Verification items for the finished model (mm, model axes). A direction names the side the tool comes from. Coordinates: 2 decimals unless noted, no trailing zeros. Write each loop counter-clockwise with the first axis right and the second up, starting at its lowest first coordinate (ties: lowest second). Pieces come first, ordered by that corner, then holes. Notation, with made-up numbers: (-2, -14.5) -> (16, -14.5) arc R16 cw to (16, 12.5) -> close; hole circle Ø3 at (-19.5, -29.5). An arc over 180 degrees is marked (long way). Write item = value, one per line. Start each with the question number.
(1) Section check B-B (y = 23). Record the cut outline in (x, z), plus the area to 3 significant figures.
(2) Material ranges on probe 1 along Z at (x, y) = (33.5, 5.5); probe 2 along Y at (x, z) = (32, 28.5); probe 3 along Z at (x, y) = (51.5, 41), recorded low to high. Write a range as [from, to].
(3) Set-up check for faces 1 (the face through (9, 35, 16)), 2 (the face through (52, 10, 16)), 3 (the face through (24.25, 5, 16)), 4 (the face through (32, 10, 24)), 5 (the face through (32, 33, 22)): record each of +Z, -Z, +X, -X, +Y, -Y from which the full face is reachable in a straight line by a thin tool's end or side.
(4) Mould release check, pull along X, two halves, no side actions. Record for faces 6 (the face through (32, 46, 24)), 7 (the face through (29.309, 4.93, 26.703)), 8 (the face through (32, 28, 0)), 9 (the face through (33, 10, 8)): released by +X, released by -X, zero draft, split by the parting line, or undercut.
(5) Gauge pin test, flat ends, axial feed: pin 1 Ø6 at (y, z) = (6, 13.5) entering from -X; pin 2 Ø3 at (y, z) = (3, 10) entering from +X; pin 3 Ø12 at (x, z) = (56.5, 16.5) entering from -Y. Record the tip position at first contact, or that the pin passes through.
(6) Section check D-D (z = 24). Record the cut outline in (x, y), plus the area to 3 significant figures.
(7) Section check C-C (x = 57.5). Record the cut outline in (y, z).
(8) Section check A-A (z = 8). Record the cut outline in (x, y).
Autodesk Inventor part; units mm, degrees
ref_plane "YZ Plane" through (0, 0, 0) normal (1, 0, 0) x (0, 1, 0)
ref_plane "XZ Plane" through (0, 0, 0) normal (0, 1, 0) x (-1, 0, 0)
ref_plane "XY Plane" through (0, 0, 0) normal (0, 0, 1) x (1, 0, 0)
sketch "Sketch1" plane through (0, 0, 0) normal (0, 0, 1) x (1, 0, 0)
  line L0 (24.25, 0) -> (39.75, 0)
  line L1 (64, 10) -> (64, 46)
  line L2 (64, 46) -> (0, 46)
  line L3 (0, 46) -> (0, 10)
  line L4 (24.25, 0) -> (24.25, 10)
  line L5 (24.25, 10) -> (0, 10)
  line L6 (39.75, 0) -> (39.75, 10)
  line L7 (39.75, 10) -> (64, 10)
  point P0 (0, 0)
  dimension "d0" = 64
  dimension "d2" = 24.25
  dimension "d3" = 10
extrude "Extrusion1" add sketch "Sketch1" along normal blind 16
sketch "Sketch2" plane through (0, 0, 16) normal (0, 0, 1) x (1, 0, 0)
  line L0 (24.25, 10) -> (24.25, 0)
  line L1 (24.25, 10) -> (24.25, 0)
  line L2 (24.25, 0) -> (39.75, 0)
  line L3 (24.25, 0) -> (39.75, 0)
  line L4 (39.75, 0) -> (39.75, 10)
  line L5 (39.75, 0) -> (39.75, 10)
  line L6 (39.75, 10) -> (64, 10)
  line L7 (39.75, 10) -> (64, 10)
  line L8 (64, 10) -> (64, 17)
  line L9 (64, 10) -> (64, 46)
  line L10 (0, 10) -> (24.25, 10)
  line L11 (0, 10) -> (0, 17)
  line L12 (0, 46) -> (0, 10)
  arc A0 (0, 17) -> (9.4683, 21.008) centre (-0.759, 31.9808) ccw
  arc A1 (54.5317, 21.008) -> (64, 17) centre (64.759, 31.9808) ccw
  line L13 (17.0879, 38.0812) -> (9.4683, 21.008)
  line L14 (46.9121, 38.0812) -> (54.5317, 21.008)
  arc A2 (46.9121, 38.0812) -> (17.0879, 38.0812) centre (32, 28) ccw
  point P0 (0, 0)
  dimension "d7" = 7
  dimension "d9" = 30
  dimension "d10" = 30
  dimension "d11" = 7
extrude "Extrusion2" add sketch "Sketch2" along normal blind 16
sketch "Sketch3" plane through (0, 0, 32) normal (0, 0, 1) x (1, 0, 0)
  circle A0 centre (32, 32.647) radius 6
  line L0 (0, 46) -> (0, 17)
  line L1 (64, 17) -> (64, 46)
  point P0 (0, 0)
  dimension "d14" = 12
  dimension "d15" = 32
  dimension "d16" = 32
extrude "Extrusion3" cut sketch "Sketch3" against normal blind 10
sketch "Sketch5" plane through (24.25, 0, 0) normal (0, -1, 0) x (1, 0, 0)
  circle A0 centre (8.0074, 24) radius 4
  circle A1 centre (8.4927, 8) radius 4
  line L0 (0, 32) -> (15.5, 32)
  line L1 (0, 0) -> (15.5, 0)
  point P0 (-24.25, 0)
  dimension "d22" = 8
  dimension "d23" = 8
  dimension "d26" = 8
  dimension "d27" = 8
extrude "Extrusion5" cut sketch "Sketch5" against normal blind 10
properties part number "pieza 4. MRKE" material "Steel, Wrought"
Response:
q1.outline = (0, 0) -> (64, 0) -> (64, 16) -> (53.64, 16) -> (53.64, 32) -> (10.36, 32) -> (10.36, 16) -> (0, 16) -> close
q1.area = 1,720 mm2
q2.probe_1 = [0, 4.07], [11.93, 20.2], [27.8, 32]
q2.probe_2 = [0, 26.65], [38.65, 46]
q2.probe_3 = [0, 16]
q3.face_1 = +Z, -X, +Y
q3.face_2 = +Z, -Z, +X, -Y
q3.face_3 = +Z, -Z, -X, -Y
q3.face_4 = -Y
q3.face_5 = +Z
q4.face_6 = split by the parting line
q4.face_7 = undercut
q4.face_8 = zero draft
q4.face_9 = undercut
q5.pin_1 = 24.25
q5.pin_2 = 39.75
q5.pin_3 = 10
q6.outline = (0, 10) -> (24.25, 10) -> (24.25, 0) -> (28.26, 0) -> (28.26, 10) -> (36.26, 10) -> (36.26, 0) -> (39.75, 0) -> (39.75, 10) -> (64, 10) -> (64, 17) arc R15 cw to (54.53, 21.01) -> (46.91, 38.08) arc R18 ccw to (17.09, 38.08) -> (9.47, 21.01) arc R15 cw to (0, 17) -> close; hole circle Ø12 at (32, 32.65)
q6.area = 1,420 mm2
q7.outline = (10, 0) -> (46, 0) -> (46, 16) -> (18.85, 16) -> (18.85, 32) -> (10, 32) -> close
q8.outline = (0, 10) -> (24.25, 10) -> (24.25, 0) -> (28.74, 0) -> (28.74, 10) -> (36.74, 10) -> (36.74, 0) -> (39.75, 0) -> (39.75, 10) -> (64, 10) -> (64, 46) -> (0, 46) -> close
